Autodesk Inventor part; units mm, degrees
ref_plane "YZ Plane" through (0, 0, 0) normal (1, 0, 0) x (0, 1, 0)
ref_plane "XZ Plane" through (0, 0, 0) normal (0, 1, 0) x (-1, 0, 0)
ref_plane "XY Plane" through (0, 0, 0) normal (0, 0, 1) x (1, 0, 0)
sketch "Sketch1" plane through (0, 0, 0) normal (0, 1, 0) x (-1, 0, 0)
  line L0 (0, 0) -> (12.7, 0)
  line L1 (12.7, 0) -> (12.7, -115.316)
  line L2 (12.7, -115.316) -> (0, -115.316)
  line L3 (0, -115.316) -> (0, 0)
  line L4 (3.175, 0) -> (9.525, 0)
  line L5 (9.525, 0) -> (9.525, 2.921)
  line L6 (9.525, 2.921) -> (3.175, 2.921)
  line L7 (3.175, 2.921) -> (3.175, 0)
  line L8 (3.175, -115.316) -> (9.525, -115.316)
  line L9 (9.525, -115.316) -> (9.525, -118.237)
  line L10 (9.525, -118.237) -> (3.175, -118.237)
  line L11 (3.175, -118.237) -> (3.175, -115.316)
  dimension "d0" = 115.316
  dimension "d1" = 12.7
  dimension "d2" = 6.35
  dimension "d3" = 3.175
  dimension "d4" = 2.921
  dimension "d5" = 2.921
  dimension "d6" = 3.175
extrude "Extrusion1" add sketch "Sketch1" along normal blind 2.921
sketch "Sketch2" plane through (0, 2.921, 0) normal (0, 1, 0) x (1, 0, 0)
  circle A0 centre (-6.35, 31.75) radius 1.5875
  circle A1 centre (-6.35, 83.566) radius 1.5875
  line L0 (0, 0) -> (0, 115.316)
  line L1 (-3.175, 0) -> (0, 0)
  line L2 (0, 115.316) -> (-3.175, 115.316)
  dimension "d9" = 3.175
  dimension "d10" = 3.175
  dimension "d11" = 6.35
  dimension "d12" = 6.35
  dimension "d13" = 31.75
  dimension "d14" = 31.75
extrude "Extrusion2" cut sketch "Sketch2" against normal blind 2.921
sketch "Sketch3" plane through (0, 2.921, 0) normal (0, 1, 0) x (1, 0, 0)
  circle A0 centre (-6.35, 57.658) radius 1.5875
  line L0 (0, 0) -> (0, 115.316)
  line L1 (-3.175, 0) -> (0, 0)
  dimension "d17" = 3.175
  dimension "d18" = 6.35
  dimension "d19" = 57.658
extrude "Extrusion3" cut sketch "Sketch3" against normal blind 2.921
sketch "Sketch4" plane through (0, 2.921, 0) normal (0, 1, 0) x (1, 0, 0)
  line L0 (0, 51.308) -> (22.225, 51.308)
  line L1 (25.4, 54.483) -> (25.4, 60.833)
  line L2 (22.225, 64.008) -> (0, 64.008)
  line L3 (0, 64.008) -> (0, 51.308)
  circle A0 centre (-6.35, 57.658) radius 1.5875
  line L4 (0, 0) -> (0, 115.316)
  circle A1 centre (19.05, 57.658) radius 1.5875
  arc A2 (25.4, 60.833) -> (22.225, 64.008) centre (22.225, 60.833) ccw
  arc A3 (22.225, 51.308) -> (25.4, 54.483) centre (22.225, 54.483) ccw
  point P0 (25.4, 64.008)
  point P1 (25.4, 51.308)
  dimension "d22" = 6.35
  dimension "d23" = 12.7
  dimension "d24" = 25.4
  dimension "d25" = 0
  dimension "d26" = 3.175
  dimension "d27" = 25.4
  dimension "d28" = 3.175
extrude "Extrusion4" add sketch "Sketch4" against normal blind 2.794 contours L3 L2 A2 L1 A3 L0
properties part number "spoonholder"
Geometry check sheet. Reference: the model listing, model coordinates, mm. A direction names the side the tool comes from. Give positions to 0.01 mm unless a question says otherwise; leave off trailing zeros. Write each loop counter-clockwise with the first axis right and the second up, starting at its lowest first coordinate (ties: lowest second). Pieces come first, ordered by that corner, then holes. Notation, with made-up numbers: M 46,-37.75 L 68,-37.75 A13 cw 68,-30.75 Z; hole C 35,-1 d10. An arc over 180 degrees is marked long. Answer as CSV lines item,"result". Start each with the question number.
Q1. Material ranges on L1, parallel to Z at x = -6.35, y = 2.2; L2, parallel to X at y = 1.7, z = -31.75; L3, parallel to Z at x = 19.05, y = 1.25, recorded low to high.
Q2. Section check C-C, the plane x = -6.35. Record the cut outline in (y, z), then the cut area to 3 significant figures.
Q3. Section check B-B, the plane z = -31.75. Record the cut outline in (x, y).
Q4. Tool access check on faces 5 (the face through (-2, 1, 0)), 6 (the face through (-3.175, 1, -117)), 7 (the face through (13, 0.127, -58)). Record the directions out of +Z, -Z, +X, -X, +Y, -Y that give a thin tool (end or side, any length) a straight path to the whole face; none if there is none.
Q5. Section check D-D, the plane y = 1.3. Give the number of separate pieces and of enclosed holes in the cut face, then the cut area to 3 significant figures.
Q6. Section check A-A, the plane x = 19.05. Record the cut outline in (y, z), then the cut area to 3 significant figures.
Q7. Go/stop test with flat-tipped pins: pin 1 (1.5 mm diameter, centred on x = -2, y = 2, fed in from -Z); pin 2 (10 mm diameter, centred on x = 16, z = -56.5, fed in from -Y); pin 3 (1 mm diameter, centred on x = 13, y = 0.5, fed in from +Z). Record where each tip stops, or that it passes through.
Q8. Release check for a two-part mould opening along X. For faces 1 (the face through (18.706, 1.544, -56.108)), 2 (the face through (-9.525, 1, -117)), 3 (the face through (-2, 1, -115.316)), 4 (the face through (-5.5, 1.48, -33.09)) record: pulls with the +X half, pulls with the -X half, needs draft (parallel to the pull), parting line crosses it, or undercut.
Geometry says:
1,L1,"-118.24 to -85.15, -81.98 to -59.25, -56.07 to -33.34, -30.16 to 2.92"
1,L2,"-12.7 to -7.94, -4.76 to 0"
1,L3,"-64.01 to -59.25, -56.07 to -51.31"
2,outline,"M 0,-118.24 L 2.92,-118.24 L 2.92,-85.15 L 0,-85.15 Z; M 0,-81.98 L 2.92,-81.98 L 2.92,-59.25 L 0,-59.25 Z; M 0,-56.07 L 2.92,-56.07 L 2.92,-33.34 L 0,-33.34 Z; M 0,-30.16 L 2.92,-30.16 L 2.92,2.92 L 0,2.92 Z"
2,area,"326 mm^2"
3,outline,"M -12.7,0 L -7.94,0 L -7.94,2.92 L -12.7,2.92 Z; M -4.76,0 L 0,0 L 0,2.92 L -4.76,2.92 Z"
4,face 5,"+Z, +X, +Y, -Y"
4,face 6,"-Z, +X, +Y, -Y"
4,face 7,"+Z, -Z, +X, -Y"
5,separate pieces,"1"
5,enclosed holes,"4"
5,area,"1,790 mm^2"
6,outline,"M 0.13,-64.01 L 2.92,-64.01 L 2.92,-59.25 L 0.13,-59.25 Z; M 0.13,-56.07 L 2.92,-56.07 L 2.92,-51.31 L 0.13,-51.31 Z"
6,area,"26.6 mm^2"
7,pin 1,"z = -115.32"
7,pin 2,"y = 0.13"
7,pin 3,"z = -51.31"
8,face 1,"undercut"
8,face 2,"pulls with the -X half"
8,face 3,"needs draft"
8,face 4,"undercut"
